from build123d import *

# Parameters (mm, degrees)
F1_DEPTH = 31.75
F3_DEPTH = 25.4
F5_DEPTH = 12.7
F7_DEPTH = 12.7
F8_DEPTH = 25.4


with BuildPart() as f1:
    # F0 (on Top) → F1 (new body)
    with BuildSketch(Plane.XY):
        Polygon((0, 37.5093027622), (0, 0), (31.75, 0), (31.75, 12.7), (69.85, 12.7), (69.85, 24.8093027622), (31.75, 24.8093027622), (31.75, 37.5093027622), align=None)
    extrude(amount=F1_DEPTH)

    # F2 (on face) → F3 (cut)
    with BuildSketch(Plane.XZ.offset(-12.7)):
        Polygon((57.15, 31.75), (69.85, 0), (69.85, 31.75), align=None)
    extrude(amount=-F3_DEPTH, mode=Mode.SUBTRACT)

    # F4 (on face) → F5 (cut)
    with BuildSketch(Plane.XZ):
        Polygon((19.05, 31.75), (31.75, 0), (31.75, 31.75), align=None)
    extrude(amount=-F5_DEPTH, mode=Mode.SUBTRACT)

    # F6 (on face) → F7 (join)
    with BuildSketch(Plane(origin=(0, 37.5093027622, 0), x_dir=(-1, 0, 0), z_dir=(0, 1, 0))):
        Polygon((-31.75, 31.75), (-31.75, 0), (-19.05, 31.75), align=None)
    extrude(amount=F7_DEPTH)

    # F8 (cut): a face of the model
    f8_faces = [f1.faces().sort_by_distance(p)[0] for p in [
        (27.5166666667, 50.2093027622, 21.1666666667),
    ]]
    extrude(f8_faces, amount=-F8_DEPTH, mode=Mode.SUBTRACT)


solid = f1.part
For this review, take the finished solid that the model builds, in its own axes (mm). A direction names the side the tool comes from. Round coordinates to 2 decimals unless told otherwise and drop trailing zeros. Order: outer loops, then holes, each group sorted by start corner. A loop starts at its lowest first (then second) coordinate and runs counter-clockwise, first axis right, second up. Notation, with made-up numbers: (29.5, -16) -> (58.5, -16) arc R25 cw to (58.5, -3) -> close; hole circle Ø1 at (24, 65.25). An arc over 180 degrees is marked (long way). Write item = value, one per line. Start each with the question number.
1) Insertion check: pin 1 (1.5 mm diameter, centred on y = 15, z = 23.5, fed in from -X); pin 2 (4 mm diameter, centred on x = 35.5, z = 7.5, fed in from -Y); pin 3 (10 mm diameter, centred on x = 38.5, y = 32, fed in from -Z); pin 4 (8 mm diameter, centred on y = 29, z = 17, fed in from +X). Each pin has a flat end and moves straight along its axis. Give the tip position at first contact, or say it passes through.
2) Take a section at B-B on x = 45. State the section outline as (y, z) points.
3) Take a section at A-A on z = 21.5. State the section outline as (x, y) points.
4) To check wall thickness, follow line 1 (Y direction, x = 49, z = 17.5); line 2 (X direction, y = 16.5, z = 25); line 3 (X direction, y = 34.5, z = 21.5). State the ranges of each line that lie inside material, in increasing order. Write a range as from..to.
5) Take a section at D-D on z = 14.5. State the section outline as (x, y) points.
6) Take a section at C-C on y = 24. State the section outline as (x, z) points.
7) Tool access review of faces 1 (the face through (44, 12.7, 16)), 2 (the face through (25.49, 31.25, 15.65)), 3 (the face through (27, 19, 0)): name each direction out of +Z, -Z, +X, -X, +Y, -Y from which nothing blocks a thin tool from reaching the whole face with its end or side.
Verdict:
q1.pin_1 = 0
q1.pin_2 = 12.7
q1.pin_3 = through
q1.pin_4 = 26.55
q2.outline = (12.7, 0) -> (24.81, 0) -> (24.81, 31.75) -> (12.7, 31.75) -> close
q3.outline = (0, 0) -> (23.15, 0) -> (23.15, 12.7) -> (61.25, 12.7) -> (61.25, 24.81) -> (23.15, 24.81) -> (23.15, 37.51) -> (0, 37.51) -> close
q4.line_1 = 12.7..24.81
q4.line_2 = 0..59.85
q4.line_3 = 0..23.15
q5.outline = (0, 0) -> (25.95, 0) -> (25.95, 12.7) -> (64.05, 12.7) -> (64.05, 24.81) -> (25.95, 24.81) -> (25.95, 37.51) -> (0, 37.51) -> close
q6.outline = (0, 0) -> (69.85, 0) -> (57.15, 31.75) -> (0, 31.75) -> close
q7.face_1 = +Z, +X, -Y
q7.face_2 = +Z, +X, +Y
q7.face_3 = -Z, +X, -X, +Y, -Y
